Read the model definition and answer for the solid it produces. Units are mm, in the model's axes. Face numbers are marked on the shaded views. A direction names the side the tool comes from. Round coordinates to 2 decimals unless told otherwise and drop trailing zeros. Order: outer loops, then holes, each group sorted by start corner. A loop starts at its lowest first (then second) coordinate and runs counter-clockwise, first axis right, second up. Notation, with made-up numbers: (46.25, 32) -> (70.25, 32) arc R22 cw to (70.25, 48) -> close; hole circle Ø9 at (-30, 51). An arc over 180 degrees is marked (long way). Answer as a JSON object with one key per item and string values. Group by question number.
Item 1: Consider probe 1 along Z at (x, y) = (48.25, 0.5) (3 decimals); probe 2 along X at (y, z) = (38, -15.1); probe 3 along Y at (x, z) = (-44.5, -1.5). Determine where each line is inside the solid, lowest interval first. Write a range as from..to.
Item 2: Section A-A, the plane x = 5 is taken. Write down the section's boundary in (y, z).
Item 3: Section B-B, the plane y = 5.5 is taken. Write down the section's boundary in (x, z).
Item 4: Section C-C, the plane z = 6 is taken. Write down the section's boundary in (x, y), plus the area to 3 significant figures.
Item 5: The mould has two halves that part along X. Classify the marked faces 4 and 5: pulls with the +X half, pulls with the -X half, needs draft (parallel to the pull), parting line crosses it, or undercut.
Item 6: For the marked faces 1, 2 and 3, determine the directions among +Z, -Z, +X, -X, +Y, -Y from which every point of the face is accessible in a straight line to the end or side of a thin tool.
Item 7: Section D-D, the plane y = 14 is taken. Write down the section's boundary in (x, z).
Item 8: Given P1, Ø1.6, axis at y = 31, z = -14.5, coming from the +X side; P2, Ø9, axis at y = 5, z = -2.5, coming from the +X side; P3, Ø8, axis at x = 46, z = -0.5, coming from the +Y side; P4, Ø12, axis at y = 10.5, z = -0.5, coming from the -X side, each flat-ended and moving along its own axis, determine where each tip first touches the part or whether it passes through.
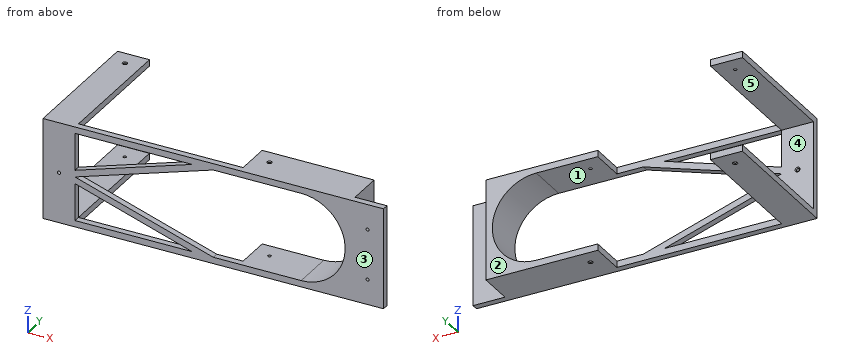
Autodesk Inventor part; units mm, degrees
ref_plane "YZ Plane" through (0, 0, 0) normal (1, 0, 0) x (0, 1, 0)
ref_plane "XZ Plane" through (0, 0, 0) normal (0, 1, 0) x (-1, 0, 0)
ref_plane "XY Plane" through (0, 0, 0) normal (0, 0, 1) x (1, 0, 0)
sketch "Эскиз1" plane through (0, 0, 0) normal (0, 1, 0) x (-1, 0, 0)
  line L0 (-53.25, 15.75) -> (53.25, 15.75)
  line L1 (53.25, 15.75) -> (53.25, -15.75)
  line L2 (53.25, -15.75) -> (-53.25, -15.75)
  line L3 (-53.25, -15.75) -> (-53.25, 15.75)
  line L4 (-53.25, 15.75) -> (53.25, -15.75) construction
  line L5 (53.25, 15.75) -> (-53.25, -15.75) construction
  line L6 (-43.25, -13.75) -> (0, -13.75)
  line L7 (43.25, -13.75) -> (43.25, -2.0986)
  line L8 (43.25, 13.75) -> (6.6012, 13.75)
  line L9 (-43.25, 13.75) -> (-43.25, -13.75)
  line L10 (0, -22.05) -> (0, 22.05) construction
  line L11 (0, -15.75) -> (0, -13.75) construction
  line L12 (0, 13.75) -> (0, 15.75) construction
  line L13 (0, -13.75) -> (43.25, 0)
  line L14 (43.25, 0) -> (0, 13.75)
  line L15 (6.6012, 13.75) -> (43.25, 2.0986)
  line L16 (43.25, -2.0986) -> (6.6012, -13.75)
  line L17 (43.25, -2.0986) -> (43.25, 2.0986) construction
  line L18 (43.25, 2.0986) -> (43.25, 13.75)
  line L19 (6.6012, -13.75) -> (43.25, -13.75)
  line L20 (0, -13.75) -> (6.6012, -13.75) construction
  line L21 (6.6012, 13.75) -> (0, 13.75) construction
  line L22 (0, 13.75) -> (-43.25, 13.75)
  line L23 (43.25, -2.0986) -> (42.644, -0.1926) construction
  line L24 (43.25, 2.0986) -> (42.644, 0.1926) construction
  point P0 (0, 0)
  point P1 (0, 0)
  dimension "d0" = 106.5
  dimension "d5" = 10
  dimension "d24" = 27.5
  dimension "d28" = 10
  dimension "d29" = 2
extrude "Выдавливание1" add sketch "Эскиз1" along normal blind 2
sketch "Эскиз2" plane through (0, 0, 0) normal (0, 1, 0) x (-1, 0, 0)
  line L0 (-43.25, -15.75) -> (-43.25, 15.75)
  line L1 (53.25, 15.75) -> (-53.25, 15.75)
  line L2 (-53.25, 15.75) -> (-53.25, -15.75)
  line L3 (0, -13.75) -> (-43.25, -13.75) construction
  line L4 (-41.25, -13.75) -> (-41.25, 13.75) construction
  line L5 (6.6012, 13.75) -> (43.25, 13.75) construction
  line L6 (-41.25, -13.75) -> (-27.5, -13.75) construction
  line L7 (-8.25, -13.75) -> (-8.25, -15.75)
  line L8 (-53.25, -15.75) -> (53.25, -15.75)
  line L9 (-8.25, -15.75) -> (-43.25, -15.75)
  line L10 (-43.25, 15.75) -> (-8.25, 15.75)
  line L11 (-8.25, 13.75) -> (-27.5, 13.75)
  line L12 (-8.25, 13.75) -> (-8.25, 15.75)
  arc A0 (-27.5, 13.75) -> (-27.5, -13.75) centre (-27.5, 0) ccw
  line L13 (-27.5, -13.75) -> (-8.25, -13.75)
  line L14 (-27.5, 13.75) -> (-41.25, 13.75) construction
  line L15 (-43.25, -13.75) -> (-43.25, 13.75)
  point P0 (0, 0)
  point P1 (43.25, -13.75)
  point P2 (-43.25, -15.75)
  dimension "d13" = 2
  dimension "d14" = 33
extrude "Выдавливание2" add sketch "Эскиз2" along normal blind 13 contours L0 L1 L12 L11 A0 L13 L7 L8
sketch "Эскиз3" plane through (0, 2, 0) normal (0, 1, 0) x (1, 0, 0)
  line L0 (-43.25, 13.75) -> (-53.25, 13.75)
  line L1 (-53.25, 13.75) -> (-53.25, 15.75)
  line L2 (-53.25, 15.75) -> (-43.25, 15.75)
  line L3 (-43.25, 15.75) -> (-43.25, 13.75)
  line L4 (-53.25, 15.75) -> (-53.25, -15.75) construction
  line L5 (-53.25, -15.75) -> (-43.25, -15.75)
  line L6 (-43.25, -15.75) -> (-43.25, -13.75)
  line L7 (-43.25, -13.75) -> (-53.25, -13.75)
  line L8 (-53.25, -13.75) -> (-53.25, -15.75)
  point P0 (0, 0)
  point P1 (8.25, -13.75)
extrude "Выдавливание3" add sketch "Эскиз3" along normal blind 41
sketch "Эскиз4" plane through (-53.25, 0, 15.75) normal (0, 0, 1) x (1, 0, 0)
  line L0 (10, 43) -> (0, 43) construction
  line L1 (0, 43) -> (10, 43) construction
  line L2 (10, 43) -> (10, 33) construction
  line L3 (10, 33) -> (0, 33) construction
  line L4 (0, 33) -> (0, 43) construction
  line L5 (106.5, 0) -> (0, 0) construction
  line L6 (0, 0) -> (0, 43) construction
  line L7 (10, 43) -> (10, 2) construction
  line L8 (10, 2) -> (61.5, 2) construction
  line L9 (61.5, 2) -> (61.5, 13) construction
  line L10 (61.5, 13) -> (96.5, 13) construction
  line L11 (96.5, 13) -> (96.5, 2) construction
  line L12 (96.5, 2) -> (106.5, 2) construction
  line L13 (106.5, 2) -> (106.5, 0) construction
  line L14 (10, 2) -> (10, 43) construction
  line L15 (0, 0) -> (0, 43) construction
  line L16 (10, 33) -> (0, 43) construction
  line L17 (10, 43) -> (0, 33) construction
  circle A0 centre (5, 38) radius 0.5
  line L18 (61.5, 13) -> (71.5, 13) construction
  line L19 (71.5, 13) -> (71.5, 3) construction
  line L20 (71.5, 3) -> (61.5, 3) construction
  line L21 (61.5, 3) -> (61.5, 13) construction
  line L22 (71.5, 13) -> (61.5, 3) construction
  line L23 (61.5, 2) -> (61.5, 13) construction
  line L24 (61.5, 13) -> (71.5, 3) construction
  circle A1 centre (66.5, 8) radius 0.5
  line L25 (0, 43) -> (10, 43)
  point P0 (53.25, 0)
  dimension "d19" = 1
  dimension "d20" = 10
  dimension "d21" = 1
hole "Отверстие1" at (-48.25, 38, 15.75) at (13.25, 8, 15.75) direction (0, 0, -1) diameter 1 depth 15.75 countersink diameter 1.5 countersink angle 90
mirror "Зеркальное отражение1" about plane through (0, 0, 0) normal (0, 0, 1) of "Отверстие1"
sketch "Эскиз5" plane through (0, 2, 0) normal (0, 1, 0) x (1, 0, 0)
  line L0 (8.25, 13.75) -> (8.25, 15.75) construction
  line L1 (-43.25, 15.75) -> (8.25, 15.75) construction
  line L2 (-53.25, 15.75) -> (-43.25, 15.75) construction
  line L3 (-53.25, 13.75) -> (-53.25, 15.75) construction
  line L4 (-43.25, 13.75) -> (-53.25, 13.75) construction
  line L5 (-43.25, 13.75) -> (-43.25, 2.0986) construction
  line L6 (-43.25, 2.0986) -> (-6.6012, 13.75) construction
  line L7 (-6.6012, 13.75) -> (-43.25, 13.75) construction
  line L8 (8.25, 13.75) -> (0, 13.75) construction
  line L9 (27.5, 13.75) -> (8.25, 13.75) construction
  arc A0 (27.5, -13.75) -> (27.5, 13.75) centre (27.5, 0) ccw construction
  line L10 (8.25, -13.75) -> (27.5, -13.75) construction
  line L11 (8.25, -15.75) -> (8.25, -13.75) construction
  line L12 (8.25, -15.75) -> (-43.25, -15.75) construction
  line L13 (-43.25, -13.75) -> (-43.25, -15.75) construction
  line L14 (-43.25, -13.75) -> (-6.6012, -13.75) construction
  line L15 (-6.6012, -13.75) -> (-43.25, -2.0986) construction
  line L16 (-43.25, -2.0986) -> (-43.25, -13.75) construction
  line L17 (8.25, 15.75) -> (43.25, 15.75) construction
  line L18 (43.25, 15.75) -> (43.25, -15.75) construction
  line L19 (53.25, -15.75) -> (43.25, -15.75) construction
  line L20 (53.25, 15.75) -> (53.25, -15.75) construction
  line L21 (43.25, 15.75) -> (53.25, 15.75) construction
  line L22 (-43.25, 15.75) -> (-43.25, 13.75) construction
  line L23 (-53.25, -13.75) -> (-53.25, 13.75) construction
  line L24 (-53.25, -15.75) -> (-53.25, -13.75) construction
  line L25 (-43.25, -15.75) -> (-53.25, -15.75) construction
  line L26 (0, 13.75) -> (-43.25, 0) construction
  line L27 (-43.25, 0) -> (0, -13.75) construction
  line L28 (0, -13.75) -> (8.25, -13.75) construction
  line L29 (43.25, -15.75) -> (8.25, -15.75) construction
  line L30 (-53.25, -13.75) -> (-43.25, -13.75) construction
  line L31 (53.25, 15.75) -> (-53.25, 15.75) construction
  line L32 (-53.25, 15.75) -> (-43.25, -15.75) construction
  line L33 (-53.25, -15.75) -> (53.25, -15.75) construction
  line L34 (-53.25, -15.75) -> (-43.25, 15.75) construction
  line L35 (53.25, 15.75) -> (43.25, 0) construction
  line L36 (43.25, 15.75) -> (53.25, 0) construction
  line L37 (53.25, -15.75) -> (53.25, 15.75) construction
  line L38 (53.25, 0) -> (43.25, -15.75) construction
  line L39 (53.25, -15.75) -> (43.25, 0) construction
  circle A1 centre (-48.25, 0) radius 0.5
  circle A2 centre (48.25, 7.875) radius 0.5
  circle A3 centre (48.25, -7.875) radius 0.5
  point P0 (0, 0)
  dimension "d37" = 1
hole "Отверстие2" at (-48.25, 2, 0) at (48.25, 2, 7.875) at (48.25, 2, -7.875) direction (0, -1, 0) diameter 1 end through all countersink diameter 1.5 countersink angle 90
properties part number "frame"
Values found:
{
 "1": {"probe 1": "-15.75..-8.375, -7.375..7.375, 8.375..15.75", "probe 2": "-53.25..-48.75, -47.75..-43.25", "probe 3": "0..2"},
 "2": {"outline": "(0, -15.75) -> (2, -15.75) -> (2, -13.75) -> (0, -13.75) -> close; (0, 13.75) -> (2, 13.75) -> (2, 15.75) -> (0, 15.75) -> close"},
 "3": {"outline": "(-53.25, -15.75) -> (-43.25, -15.75) -> (-43.25, -13.75) -> (-53.25, -13.75) -> close; (-53.25, 13.75) -> (-43.25, 13.75) -> (-43.25, 15.75) -> (-53.25, 15.75) -> close; (8.25, -15.75) -> (43.25, -15.75) -> (43.25, 15.75) -> (8.25, 15.75) -> (8.25, 13.75) -> (27.5, 13.75) arc R13.75 cw to (27.5, -13.75) -> (8.25, -13.75) -> close"},
 "4": {"outline": "(-53.25, 0) -> (-43.25, 0) -> (-43.25, 2) -> (-53.25, 2) -> close; (-30.98, 0) -> (-24.38, 0) -> (-24.38, 2) -> (-30.98, 2) -> close; (39.87, 0) -> (53.25, 0) -> (53.25, 2) -> (43.25, 2) -> (43.25, 13) -> (39.87, 13) -> close", "area": "97.1 mm2"},
 "5": {"face 4": "undercut", "face 5": "needs draft"},
 "6": {"face 1": "+Y, -Y", "face 2": "+Z, -Z, +X, +Y", "face 3": "+Z, -Z, +X, -X, -Y"},
 "7": {"outline": "(-53.25, -15.75) -> (-43.25, -15.75) -> (-43.25, -13.75) -> (-53.25, -13.75) -> close; (-53.25, 13.75) -> (-43.25, 13.75) -> (-43.25, 15.75) -> (-53.25, 15.75) -> close"},
 "8": {"P1": "x = -43.25", "P2": "x = 53.25", "P3": "y = 13", "P4": "x = 39.62"}
}
